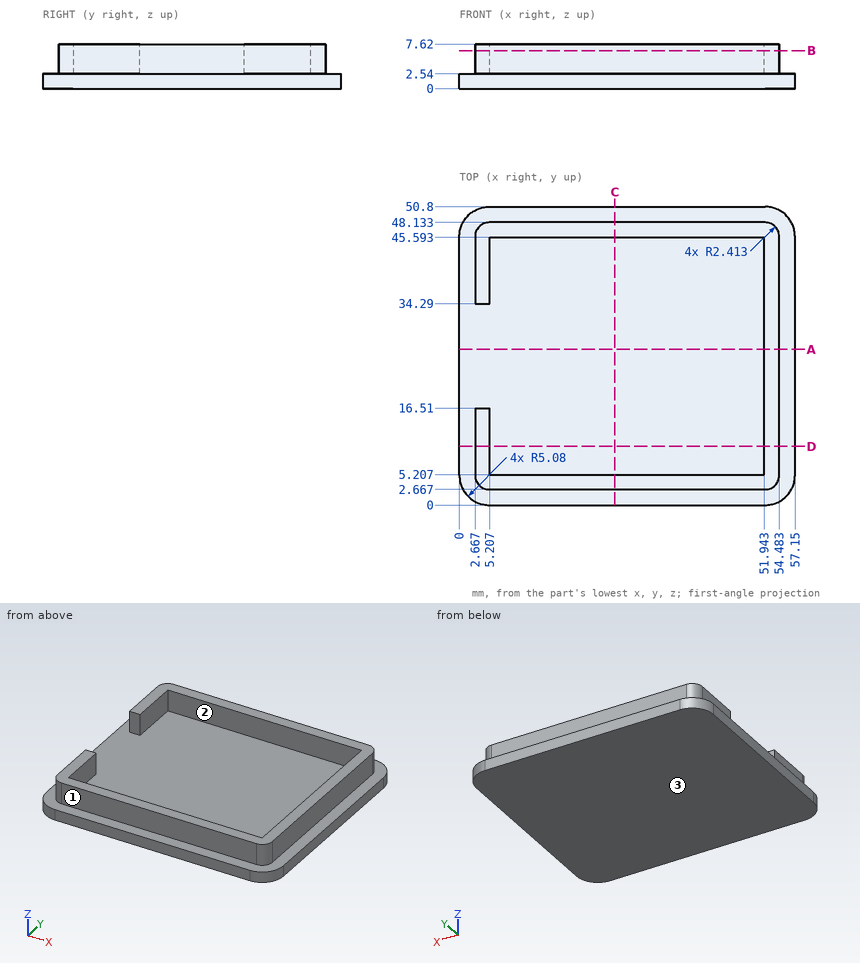
Could you check a few things on this drawing? It's one solid part, dimensions in mm from its lowest x, y, z. Coordinates: 2 decimals unless noted, no trailing zeros. Order: outer loops, then holes, each group sorted by start corner. A loop starts at its lowest first (then second) coordinate and runs counter-clockwise, first axis right, second up. Notation, with made-up numbers: M 52.5,-27 L 83.5,-27 A13 cw 83.5,-20 Z; hole C 70.5,70.25 d11. An arc over 180 degrees is marked long. Use a Markdown table: item, result. Add a question column.
Q1. We'd pull the mould along Y, two halves only. Please class the marked faces 1, 2 and 3: pulls with the +Y half, pulls with the -Y half, needs draft (parallel to the pull), parting line crosses it, or undercut.
Q2. I want a section at C-C on x = 26.5. List the corners of the cut face in (y, z) for me, then the cut area to 3 significant figures.
Q3. I want a section at A-A on y = 26.5. List the corners of the cut face in (x, z) for me.
Q4. I'm going to push flat-ended pins straight in: pin 1 (1 mm diameter, centred on x = 20, y = 8, fed in from +Z); pin 2 (2 mm diameter, centred on x = 3.5, z = 5, fed in from -Y); pin 3 (2.5 mm diameter, centred on y = 9.5, z = 5, fed in from +X). Where does each tip first touch, or does it pass through?
Q5. I want a section at D-D on y = 10. List the corners of the cut face in (x, z) for me, then the cut area to 3 significant figures.
Q6. If I drill on L1, parallel to Y at x = 30, z = 5.5; L2, parallel to X at y = 45, z = 5.5; L3, parallel to Z at x = 48, y = 6.5, over which ranges is the centre line in solid material (lowest first)?
Q7. I want a section at B-B on z = 6.5. List the corners of the cut face in (x, y) for me, then the cut area to 3 significant figures.
Checked values:
| question | item | result |
|---|---|---|
| 1 | face 1 | pulls with the -Y half |
| 1 | face 2 | undercut |
| 1 | face 3 | needs draft |
| 2 | outline | M 0,0 L 50.8,0 L 50.8,2.54 L 48.13,2.54 L 48.13,7.62 L 45.59,7.62 L 45.59,2.54 L 5.21,2.54 L 5.21,7.62 L 2.67,7.62 L 2.67,2.54 L 0,2.54 Z |
| 2 | area | 155 mm² |
| 3 | outline | M 0,0 L 57.15,0 L 57.15,2.54 L 54.48,2.54 L 54.48,7.62 L 51.94,7.62 L 51.94,2.54 L 0,2.54 Z |
| 4 | pin 1 | z = 2.54 |
| 4 | pin 2 | y = 2.74 |
| 4 | pin 3 | x = 54.48 |
| 5 | outline | M 0,0 L 57.15,0 L 57.15,2.54 L 54.48,2.54 L 54.48,7.62 L 51.94,7.62 L 51.94,2.54 L 5.21,2.54 L 5.21,7.62 L 2.67,7.62 L 2.67,2.54 L 0,2.54 Z |
| 5 | area | 171 mm² |
| 6 | L1 | 2.67 to 5.21, 45.59 to 48.13 |
| 6 | L2 | 2.67 to 5.21, 51.94 to 54.48 |
| 6 | L3 | 0 to 2.54 |
| 7 | outline | M 2.67,5.08 A2.41 ccw 5.08,2.67 L 52.07,2.67 A2.41 ccw 54.48,5.08 L 54.48,45.72 A2.41 ccw 52.07,48.13 L 5.08,48.13 A2.41 ccw 2.67,45.72 L 2.67,34.29 L 5.21,34.29 L 5.21,45.59 L 51.94,45.59 L 51.94,5.21 L 5.21,5.21 L 5.21,16.51 L 2.67,16.51 Z |
| 7 | area | 418 mm² |
